Read the model definition and answer for the solid it produces. Units are mm, in the model's axes. A direction names the side the tool comes from. Give positions to 0.01 mm unless a question says otherwise; leave off trailing zeros. Write each loop counter-clockwise with the first axis right and the second up, starting at its lowest first coordinate (ties: lowest second). Pieces come first, ordered by that corner, then holes. Notation, with made-up numbers: M 14,13 L 63,13 A8 cw 63,22 Z; hole C 48.5,47.25 d3. An arc over 180 degrees is marked long. Put each result on its own line as item: value.
from build123d import *

# Parameters (mm, degrees)
F0_W     = 95.25
F0_H     = 69.85
F0_W_2   = 82.55
F0_H_2   = 57.15
F1_DEPTH = 2.794
F0_W_3   = 77.174016
F0_H_3   = 51.943318
F2_DEPTH = 5.334
F0_W_4   = 63.5
F0_H_4   = 25.4
F3_DEPTH = 2.794


with BuildPart() as f1:
    # F0 (on Top) → F1 (new body)
    with BuildSketch(Plane.XY):
        Rectangle(F0_W, F0_H)
        Rectangle(F0_W_2, F0_H_2, mode=Mode.SUBTRACT)
    extrude(amount=F1_DEPTH)

    # F0 (on Top) → F2 (join)
    with BuildSketch(Plane.XY):
        Rectangle(F0_W_2, F0_H_2)
        Rectangle(F0_W_3, F0_H_3, mode=Mode.SUBTRACT)
    extrude(amount=F2_DEPTH)

    # F0 (on Top) → F3 (join)
    with BuildSketch(Plane.XY):
        Rectangle(F0_W_3, F0_H_3)
        Rectangle(F0_W_4, F0_H_4, mode=Mode.SUBTRACT)
    extrude(amount=F3_DEPTH)


solid = f1.part
(1) Straight lines are drawn through the part: line 1 along X through (y, z) = (-21, 3.25) (3 decimals); line 2 along Y through (x, z) = (-14, 1.1) (3 decimals); line 3 along Y through (x, z) = (-16, 3.85) (3 decimals). For each, find the intervals that lie inside material, in ascending order. Write a range as from..to.
Result:
line 1: x = -41.275..-38.587, 38.587..41.275
line 2: y = -34.925..-12.7, 12.7..34.925
line 3: y = -28.575..-25.972, 25.972..28.575
(2) For a pull along Y with two mould halves and no side action, classify faces 6 (the face through (-38.587, 0, 4)), 7 (the face through (-1, -34.925, 1)), 8 (the face through (-1, 34.925, 1)) as +Y half, -Y half, draft (parallel to the pull), parting line (faces both ways), or undercut.
Result:
face 6: undercut
face 7: -Y half
face 8: +Y half
(3) Which of the six approach directions +Z, -Z, +X, -X, +Y, -Y give full straight-line access (tool end or side, diameter ignored) to faces 1 (the face through (41.275, 0, 4)), 2 (the face through (0, -12.7, 1)), 3 (the face through (-41.275, 0, 4)), 4 (the face through (-1, 28.575, 4)), 5 (the face through (-1, 18, 2.794))?
Result:
face 1: +Z, +X, +Y, -Y
face 2: +Z, -Z
face 3: +Z, -X, +Y, -Y
face 4: +Z, +X, -X, +Y
face 5: +Z
(4) Section B-B on y = 10 is taken. Determine the outline of the cut face in (x, z) (3 decimals).
Result:
outline: M -47.625,0 L -31.75,0 L -31.75,2.794 L -38.587,2.794 L -38.587,5.334 L -41.275,5.334 L -41.275,2.794 L -47.625,2.794 Z; M 31.75,0 L 47.625,0 L 47.625,2.794 L 41.275,2.794 L 41.275,5.334 L 38.587,5.334 L 38.587,2.794 L 31.75,2.794 Z
(5) Given pin 1 Ø3 at (y, z) = (-22.5, 4.5) entering from +X (3 decimals); pin 2 Ø1.3 at (x, z) = (-12, 3.5) entering from +Y (3 decimals); pin 3 Ø2 at (x, z) = (17.5, 4.5) entering from -Y (3 decimals), each flat-ended and moving along its own axis, determine where each tip first touches the part or whether it passes through.
Result:
pin 1: stops at x = 41.275
pin 2: stops at y = 28.575
pin 3: stops at y = -28.575
(6) Section D-D on y = -20 is taken. Determine the outline of the cut face in (x, z) (3 decimals).
Result:
outline: M -47.625,0 L 47.625,0 L 47.625,2.794 L 41.275,2.794 L 41.275,5.334 L 38.587,5.334 L 38.587,2.794 L -38.587,2.794 L -38.587,5.334 L -41.275,5.334 L -41.275,2.794 L -47.625,2.794 Z
(7) Section C-C on x = -18 is taken. Determine the outline of the cut face in (y, z) (3 decimals).
Result:
outline: M -34.925,0 L -12.7,0 L -12.7,2.794 L -25.972,2.794 L -25.972,5.334 L -28.575,5.334 L -28.575,2.794 L -34.925,2.794 Z; M 12.7,0 L 34.925,0 L 34.925,2.794 L 28.575,2.794 L 28.575,5.334 L 25.972,5.334 L 25.972,2.794 L 12.7,2.794 Z
(8) Section A-A on z = 3.8 is taken. Determine the outline of the cut face in (x, y) (3 decimals), and give its area (3 significant figures).
Result:
outline: M -41.275,-28.575 L 41.275,-28.575 L 41.275,28.575 L -41.275,28.575 Z; hole M -38.587,-25.972 L 38.587,-25.972 L 38.587,25.972 L -38.587,25.972 Z
area: 709 mm²
